Autodesk Inventor part; units mm, degrees
ref_plane "YZ Plane" through (0, 0, 0) normal (1, 0, 0) x (0, 1, 0)
ref_plane "XZ Plane" through (0, 0, 0) normal (0, 1, 0) x (-1, 0, 0)
ref_plane "XY Plane" through (0, 0, 0) normal (0, 0, 1) x (1, 0, 0)
sketch "Sketch1" plane through (0, 0, 0) normal (0, 0, 1) x (1, 0, 0)
  line L0 (0.65, -95.0088) -> (0.65, -83.2008) construction
  line L1 (2.65, -83.2008) -> (2.65, -91.0088) construction
  line L2 (2.65, -91.0088) -> (4.65, -91.0088) construction
  line L3 (4.65, -91.0088) -> (0.65, -95.0088) construction
  circle A0 centre (15.35, -55.1458) radius 14.7 construction
  line L4 (3.0006, -90.8088) -> (30.45, -86.6259)
  line L5 (30.45, -86.6259) -> (30.2994, -85.6374)
  line L6 (30.2994, -85.6374) -> (2.85, -89.8202)
  line L7 (2.85, -89.8202) -> (3.0006, -90.8088)
  line L8 (30.45, -86.6259) -> (30.45, -70.1877) construction
  line L9 (25.65, -86.3458) -> (5.15, -86.3458)
  line L10 (5.15, -86.3458) -> (5.15, -69.8458)
  line L11 (25.65, -69.8458) -> (5.15, -69.8458)
  line L12 (25.65, -86.3458) -> (25.65, -69.8458)
  line L13 (0.65, -83.2008) -> (2.65, -83.2008)
  dimension "d0" = 1
  dimension "d1" = 0.2
  dimension "d2" = 0.2
  dimension "d3" = 0.4
  dimension "d4" = 0
  dimension "d17" = 27.7662
extrude "Extrusion1" [suppressed]
sketch "Sketch2" plane through (30.45, -86.6259, -50) normal (0.1506, -0.9886, 0) x (0.9886, 0.1506, 0)
  line L0 (-25.9454, 16.5) -> (-25.9454, 83.5)
  line L1 (-27.9685, 0) -> (-27.9685, 3)
  circle A0 centre (-5.2783, 96.6469) radius 1.5
  circle A1 centre (-14.8697, 96.6469) radius 1.5
  circle A2 centre (-14.8697, 3.3531) radius 1.5
  circle A3 centre (-5.2783, 3.3531) radius 1.5
  circle A4 centre (-9.5918, 90.5) radius 4
  circle A5 centre (-20.1476, 90.5) radius 4
  circle A6 centre (-9.5918, 9.5) radius 4
  circle A7 centre (-20.1476, 9.5) radius 4
  line L2 (-27.3313, 20) -> (-27.3313, 3)
  line L3 (-2.2753, 15.5) -> (-24.9339, 15.5)
  line L4 (-13.8886, 7.2533) -> (-16.5988, 7.2533)
  line L5 (-27.9685, 20) -> (-27.9685, 80)
  line L6 (-2.2753, 3.6302) -> (-2.2753, 0)
  arc A8 (-7.1381, 5.9818) -> (-2.2753, 3.6302) centre (-5.2753, 3.6302) ccw
  arc A9 (-2.2753, 3.6302) -> (-7.1381, 5.9818) centre (-5.2753, 3.6302) ccw
  line L7 (-2.2753, 15.5) -> (-2.2753, 3.6302)
  line L8 (-27.3313, 3) -> (-27.9685, 3)
  ellipse E0 centre (-20.5244, 90.5) end of major axis (-15.9938, 90.5) minor radius 4.5 (-16.5988, 92.7467) -> (-16.5988, 88.2533) ccw
  line L9 (-16.5988, 92.7467) -> (-13.8886, 92.7467)
  ellipse E1 centre (-9.963, 90.5) end of major axis (-5.4324, 90.5) minor radius 4.5 (-7.1381, 94.0182) -> (-13.8886, 92.7467) ccw
  arc A10 (-2.2753, 96.3698) -> (-7.1381, 94.0182) centre (-5.2753, 96.3698) ccw
  line L10 (-2.2753, 96.3698) -> (-2.2753, 100)
  line L11 (-2.2753, 100) -> (-27.9685, 100)
  line L12 (-27.9685, 97) -> (-27.9685, 100)
  line L13 (-27.9685, 97) -> (-27.3313, 97)
  line L14 (-27.3313, 97) -> (-27.3313, 80)
  line L15 (-27.3313, 80) -> (-27.9685, 80)
  ellipse E2 centre (-24.9339, 83.5) end of major axis (-25.9454, 83.5) minor radius 1 (-24.9339, 84.5) -> (-25.9454, 83.5) ccw
  line L16 (-2.2753, 84.5) -> (-24.9339, 84.5)
  line L17 (-2.2753, 84.5) -> (-2.2753, 96.3698)
  arc A11 (-7.1381, 94.0182) -> (-2.2753, 96.3698) centre (-5.2753, 96.3698) ccw
  ellipse E3 centre (-9.963, 90.5) end of major axis (-5.4324, 90.5) minor radius 4.5 (-13.8886, 88.2533) -> (-7.1381, 94.0182) ccw
  line L18 (-13.8886, 88.2533) -> (-16.5988, 88.2533)
  circle A12 centre (-15.2437, 96.3698) radius 3
  ellipse E4 centre (-9.963, 9.5) end of major axis (-5.4324, 9.5) minor radius 4.5 (-13.8886, 7.2533) -> (-7.1381, 5.9818) ccw
  ellipse E5 centre (-9.963, 9.5) end of major axis (-5.4324, 9.5) minor radius 4.5 (-7.1381, 5.9818) -> (-13.8886, 11.7467) ccw
  circle A13 centre (-15.2437, 3.6302) radius 3
  line L19 (-27.9685, 20) -> (-27.3313, 20)
  line L20 (-2.2753, 0) -> (-27.9685, 0)
  ellipse E6 centre (-20.5244, 9.5) end of major axis (-15.9938, 9.5) minor radius 4.5 (-16.5988, 11.7467) -> (-16.5988, 7.2533) ccw
  line L21 (-16.5988, 11.7467) -> (-13.8886, 11.7467)
  ellipse E7 centre (-24.9339, 16.5) end of major axis (-25.9454, 16.5) minor radius 1 (-25.9454, 16.5) -> (-24.9339, 15.5) ccw
  point P0 (-17.0528, 50)
  point P1 (-16.268, 7.2533)
  point P2 (-16.3079, 7.2533)
  point P3 (-16.3688, 7.2533)
  point P4 (-16.5217, 7.2533)
  point P5 (-16.5463, 7.2533)
  point P6 (-14.6243, 7.2533)
  point P7 (-17.1998, 7.2533)
  point P8 (-9.892, 13.95)
  point P9 (-28.626, 82.5)
  point P10 (-14.5461, 11.7467)
  dimension "d7" = 3
  dimension "d8" = 3
  dimension "d9" = 3
  dimension "d10" = 3
  dimension "d13" = 8
  dimension "d14" = 8
  dimension "d15" = 8
  dimension "d16" = 8
extrude "Extrusion2" [suppressed]
sketch "Sketch5" plane through (0, 0, 0) normal (0, 1, 0) x (-1, 0, 0)
  line L0 (0, -100) -> (0, 0)
  line L1 (0, 0) -> (-26.4787, 0)
  line L2 (-26.4787, 0) -> (-26.4787, -100)
  line L3 (-26.4787, -100) -> (0, -100)
  circle A0 centre (-6.2585, -9.5) radius 4
  circle A1 centre (-21.2257, -96.6288) radius 1.5
  circle A2 centre (-11.5653, -3.3712) radius 1.5
  circle A3 centre (-16.8722, -90.5) radius 4
  circle A4 centre (-16.8722, -9.5) radius 4
  circle A5 centre (-11.5653, -96.6288) radius 1.5
  circle A6 centre (-21.2257, -3.3712) radius 1.5
  circle A7 centre (-6.2585, -90.5) radius 4
  point P0 (0, 0)
  dimension "d2" = 0.2
extrude "Extrusion5" add sketch "Sketch5" against normal blind 1
equation "\"d14\" = d13"
equation "\"d15\" = d13"
equation "\"d16\" = d13"
properties part number "SteelFront" material "Steel, Alloy"
Design review of the part built by this model. Coordinates are the model's own, in mm. Round coordinates to 2 decimals unless told otherwise and drop trailing zeros. Loops run counter-clockwise (first coordinate to the right, second up) from the corner with the lowest first, then second, coordinate; pieces in that order, holes last. Notation, with made-up numbers: (-0.75, 50.5) - (12.25, 50.5) arc R9 cw to (12.25, 55.5) - close; hole circle Ø10 at (-7.5, 7.25). An arc over 180 degrees is marked (long way). One line per item, written item: value. Start each with the question number.
1) Consider section A-A on z = -9.5. Give the boundary of the cut face in (x, y), then the cut area to 3 significant figures.
2) Consider section C-C on z = -92. Give the boundary of the cut face in (x, y), then the cut area to 3 significant figures.
3) Draft analysis for pull direction X (two halves, no side actions). For faces 1 (the flat face through (13, -1, -49)), 2 (the cylindrical face through (22.724, -0.493, -3.305)), state which applies: +X half, -X half, draft (parallel to the pull), parting line (faces both ways), or undercut.
4) To check wall thickness, follow L1, parallel to Z at x = 6, y = -0.2; L2, parallel to Z at x = 3, y = -0.15; L3, parallel to X at y = -0.85, z = -92.5. State the ranges of each line that lie inside material, in increasing order. Write a range as from..to.
5) Consider section B-B on y = -0.8. Give the number of separate pieces and of enclosed holes in the cut face, then the cut area to 3 significant figures.
Reported:
1. outline: (0, -1) - (2.26, -1) - (2.26, 0) - (0, 0) - close; (10.26, -1) - (12.87, -1) - (12.87, 0) - (10.26, 0) - close; (20.87, -1) - (26.48, -1) - (26.48, 0) - (20.87, 0) - close
1. area: 10.5 mm^2
2. outline: (0, -1) - (2.55, -1) - (2.55, 0) - (0, 0) - close; (9.97, -1) - (13.16, -1) - (13.16, 0) - (9.97, 0) - close; (20.58, -1) - (26.48, -1) - (26.48, 0) - (20.58, 0) - close
2. area: 11.6 mm^2
3. face 1: draft
3. face 2: undercut
4. L1: z = -100..-94.49, -86.51..-13.49, -5.51..0
4. L2: z = -100..-92.82, -88.18..-11.82, -7.18..0
4. L3: x = 0..2.79, 9.72..13.41, 20.34..26.48
5. separate pieces: 1
5. enclosed holes: 8
5. area: 2,420 mm^2
